The listing builds one solid part. Answer for the finished solid, in the listing's coordinates (mm). A direction names the side the tool comes from. Round coordinates to 2 decimals unless told otherwise and drop trailing zeros. Loops run counter-clockwise (first coordinate to the right, second up) from the corner with the lowest first, then second, coordinate; pieces in that order, holes last. Notation, with made-up numbers: (40, -17.5) - (51, -17.5) arc R36 ccw to (51, 16.5) - close; hole circle Ø1 at (56, 50.25). An arc over 180 degrees is marked (long way). Write item = value, one per line. Start each with the question number.
1) Straight lines are drawn through the part: line 1 along Y through (x, z) = (0, 1.6); line 2 along Y through (x, z) = (-5, 2); line 3 along X through (y, z) = (-12, 0.75). For each, find the intervals that lie inside material, in ascending order.
2) Given pin 1 Ø0.8 at (y, z) = (-12, 1) entering from -X; pin 2 Ø0.8 at (y, z) = (-11.5, 1.5) entering from +X; pin 3 Ø5.5 at (x, y) = (0, 0) entering from +Z; pin 4 Ø1.5 at (x, z) = (7, 1) entering from +Y, each flat-ended and moving along its own axis, determine where each tip first touches the part or whether it passes through.
3) A tool of negligible diameter and unlimited length cuts with its end or side. For faces 1 (the flat face through (-4, 57, 1)), 2 (the cylindrical face through (4.326, 5.212, 1.257)), 3 (the flat face through (0, 75, 0)), 4 (the flat face through (-1, -12, 1)), from which of +Z, -Z, +X, -X, +Y, -Y can it reach the whole face along a straight path? Write none if from no direction.
4) Section C-C, the plane y = 116 is taken. Determine the outline of the cut face in (x, z).
5) For a pull along Y with two mould halves and no side action, classify faces 5 (the cylindrical face through (0, 132, 1)), 6 (the flat face through (4, -11, 1)), 7 (the cylindrical face through (6.075, 127.686, 1.257)), 8 (the cylindrical face through (-4.326, -5.212, 1.257)) as released by +Y, released by -Y, zero draft, split by the parting line, or undercut.
6) Section A-A, the plane z = 1.1 is taken. Give the number of separate pieces and of enclosed holes in the cut face, and give its area (3 significant figures).
7) Section B-B, the plane y = 0 is taken. Determine the outline of the cut face in (x, z).
8) Section D-D, the plane y = 35 is taken. Determine the outline of the cut face in (x, z).
from build123d import *

# Parameters (mm, degrees)
MODEL_R             = 3.55
MODEL_R_2           = 2
BOSS_EXTRUDE1_DEPTH = 2.55


with BuildPart() as part:
    # Model → Boss-Extrude1 (new body)
    with BuildSketch(Plane.XY):
        with BuildLine():
            Line((-4, 105.347524158), (-4, 7.745966692))
            ThreePointArc((-4, 7.745966692), (-4.317541634, 5.245966692), (-5.25, 2.90473751))
            ThreePointArc((-5.25, 2.90473751), (-6, 0), (-5.25, -2.90473751))
            ThreePointArc((-5.25, -2.90473751), (-4.317541634, -5.245966692), (-4, -7.745966692))
            Line((-4, -7.745966692), (-4, -13.8))
            ThreePointArc((-4, -13.8), (0, -17.8), (4, -13.8))
            Line((4, -13.8), (4, -7.745966692))
            ThreePointArc((4, -7.745966692), (4.317541634, -5.245966692), (5.25, -2.90473751))
            ThreePointArc((5.25, -2.90473751), (6, 0), (5.25, 2.90473751))
            ThreePointArc((5.25, 2.90473751), (4.317541634, 5.245966692), (4, 7.745966692))
            Line((4, 7.745966692), (4, 105.347524158))
            ThreePointArc((4, 105.347524158), (4.871290708, 109.430007062), (7.333333333, 112.801084083))
            ThreePointArc((7.333333333, 112.801084083), (0, 132), (-7.333333333, 112.801084083))
            ThreePointArc((-7.333333333, 112.801084083), (-4.871290708, 109.430007062), (-4, 105.347524158))
        make_face()
        Circle(MODEL_R, mode=Mode.SUBTRACT)
        with Locations((0, 121)):
            Circle(MODEL_R_2, mode=Mode.SUBTRACT)
        with Locations((-5, 126)):
            Circle(MODEL_R_2, mode=Mode.SUBTRACT)
        with Locations((5, 126)):
            Circle(MODEL_R_2, mode=Mode.SUBTRACT)
        with Locations((5, 116)):
            Circle(MODEL_R_2, mode=Mode.SUBTRACT)
        with Locations((-5, 116)):
            Circle(MODEL_R_2, mode=Mode.SUBTRACT)
        with BuildLine():
            Line((-1, -10.1), (-1, -13.8))
            ThreePointArc((-1, -13.8), (0, -14.8), (1, -13.8))
            Line((1, -13.8), (1, -10.1))
            ThreePointArc((1, -10.1), (0, -9.1), (-1, -10.1))
        make_face(mode=Mode.SUBTRACT)
        with BuildLine():
            Line((-1, 15.1), (-1, 10.1))
            ThreePointArc((-1, 10.1), (0, 9.1), (1, 10.1))
            Line((1, 10.1), (1, 15.1))
            ThreePointArc((1, 15.1), (0, 16.1), (-1, 15.1))
        make_face(mode=Mode.SUBTRACT)
    extrude(amount=BOSS_EXTRUDE1_DEPTH)


solid = part.part
Geometry check:
q1.line_1 = -17.8 to -14.8, -9.1 to -3.55, 3.55 to 9.1, 16.1 to 119, 123 to 132
q1.line_2 = -3.39 to 3.39, 109.71 to 114, 118 to 124, 128 to 130.8
q1.line_3 = -4 to -1, 1 to 4
q2.pin_1 = -4
q2.pin_2 = 4
q2.pin_3 = through
q2.pin_4 = 130.05
q3.face_1 = +Z, -Z, -X
q3.face_2 = +Z, -Z, +X
q3.face_3 = -Z, +X, -X, +Y, -Y
q3.face_4 = +Z, -Z
q4.outline = (-9.8, 0) - (-7, 0) - (-7, 2.55) - (-9.8, 2.55) - close; (-3, 0) - (3, 0) - (3, 2.55) - (-3, 2.55) - close; (7, 0) - (9.8, 0) - (9.8, 2.55) - (7, 2.55) - close
q5.face_5 = split by the parting line
q5.face_6 = zero draft
q5.face_7 = undercut
q5.face_8 = released by -Y
q6.separate_pieces = 1
q6.enclosed_holes = 8
q6.area = 1,310 mm2
q7.outline = (-6, 0) - (-3.55, 0) - (-3.55, 2.55) - (-6, 2.55) - close; (3.55, 0) - (6, 0) - (6, 2.55) - (3.55, 2.55) - close
q8.outline = (-4, 0) - (4, 0) - (4, 2.55) - (-4, 2.55) - close
